from build123d import *

# Parameters (mm, degrees)
F0_R     = 47.425986
F1_DEPTH = 25.4
F2_R     = 35.341505
F3_DEPTH = 22.352
F4_R     = 27.718255
F5_DEPTH = 14.224
F6_R     = 15.158749
F7_DEPTH = 68.326


with BuildPart() as f1:
    # F0 (on Top) → F1 (new body)
    with BuildSketch(Plane.XY):
        Circle(F0_R)
    extrude(amount=F1_DEPTH)

    # F2 (on Top) → F3 (join)
    with BuildSketch(Plane.XY):
        Circle(F2_R)
    extrude(amount=-F3_DEPTH)

    # F4 (on face) → F5 (join)
    with BuildSketch(Plane(origin=(0, 0, -22.352), x_dir=(1, 0, 0), z_dir=(0, 0, -1))):
        Circle(F4_R)
    extrude(amount=F5_DEPTH)

    # F6 (on Top) → F7 (join)
    with BuildSketch(Plane.XY):
        Circle(F6_R)
    extrude(amount=-F7_DEPTH)


solid = f1.part
Here's how the part is built. I have some questions about the finished solid (model axes, mm). A direction names the side the tool comes from. Round coordinates to 2 decimals unless told otherwise and drop trailing zeros. Write each loop counter-clockwise with the first axis right and the second up, starting at its lowest first coordinate (ties: lowest second). Pieces come first, ordered by that corner, then holes.
1. Suppose I cut it at A-A (y = 0). List the corners of the cut face in (x, z) for me.
2. For faces 1 (the cylindrical face through (-6.174, 47.022, 12.522)), 2 (the cylindrical face through (-1.97, 15.03, -52.23)), which set-ups out of +Z, -Z, +X, -X, +Y, -Y let a thin tool reach every point of the face, with its end or its side?
3. Suppose I cut it at C-C (z = 15.5). List the corners of the cut face in (x, y) for me.
4. Will these pins go through, and if not, where does the flat tip stop? pin 1 Ø8 at (y, z) = (6, -22.5) entering from -X; pin 2 Ø6 at (y, z) = (37.5, 14) entering from -X; pin 3 Ø3 at (x, y) = (-28.5, 12) entering from -Z.
5. I need wall thicknesses on L1, parallel to Z at x = -20, y = -33; L2, parallel to Z at x = -26.5, y = -11; L3, parallel to X at y = 24, z = 21.5. Which ranges of each line are inside material? Lowest first, please.
6. Suppose I cut it at D-D (x = -24). List the corners of the cut face in (y, z) for me.
Answer sheet:
1. outline: (-47.43, 0) - (-35.34, 0) - (-35.34, -22.35) - (-27.72, -22.35) - (-27.72, -36.58) - (-15.16, -36.58) - (-15.16, -68.33) - (15.16, -68.33) - (15.16, -36.58) - (27.72, -36.58) - (27.72, -22.35) - (35.34, -22.35) - (35.34, 0) - (47.43, 0) - (47.43, 25.4) - (-47.43, 25.4) - close
2. face 1: +Z, -Z
2. face 2: -Z
3. outline: circle Ø94.85 at (0, 0)
4. pin 1: stops at x = -35.28
4. pin 2: stops at x = -32.54
4. pin 3: stops at z = -22.35
5. L1: z = 0 to 25.4
5. L2: z = -22.35 to 25.4
5. L3: x = -40.91 to 40.91
6. outline: (-40.91, 0) - (-25.94, 0) - (-25.94, -22.35) - (-13.87, -22.35) - (-13.87, -36.58) - (13.87, -36.58) - (13.87, -22.35) - (25.94, -22.35) - (25.94, 0) - (40.91, 0) - (40.91, 25.4) - (-40.91, 25.4) - close
